from build123d import *

# Parameters (mm, degrees)
EXTRUDE004_DEPTH                     = 120
EXTRUDE004_ONTO_SKETCH004_ROLL_ANGLE = 90
ARRAY005_X_COUNT                     = 2
ARRAY005_X_PITCH                     = 51
EXTRUDE001_DEPTH                     = 120
EXTRUDE001_ONTO_SKETCH001_ROLL_ANGLE = 90
ARRAY003_Z_COUNT                     = 2
ARRAY003_Z_PITCH                     = 21
EXTRUDE003_DEPTH                     = 119
EXTRUDE003_ONTO_SKETCH003_ROLL_ANGLE = 90
ARRAY_X_COUNT                        = 2
ARRAY_X_PITCH                        = 51
EXTRUDE002_DEPTH                     = 119
EXTRUDE002_ONTO_SKETCH002_ROLL_ANGLE = 90
ARRAY004_Z_COUNT                     = 2
ARRAY004_Z_PITCH                     = 21
BOX002_W                             = 96
BOX002_H                             = 118
BOX002_DEPTH                         = 1
BOX001_W                             = 96
BOX001_H                             = 118
BOX001_DEPTH                         = 41
BOX_W                                = 102
BOX_H                                = 120
BOX_DEPTH                            = 47
EXTRUDE_DEPTH                        = 0.8
ARRAY002_X_COUNT                     = 8
ARRAY002_X_PITCH                     = 12
ARRAY002_Z_COUNT                     = 2
ARRAY002_Z_PITCH                     = 21
FILLET_R                             = 0.5


with BuildPart() as bottomsideguidearray:
    # Sketch004 as drawn → Extrude004 (new)
    with BuildSketch(Plane.XY):
        Polygon((-6, 1), (4, 1), (2, -1), (-4, -1), align=None)
    extrude(amount=-EXTRUDE004_DEPTH)


with BuildPart() as bottomsideguidearray_1:
    # Extrude004 onto Sketch004 roll: moved
    add(bottomsideguidearray.part.rotate(Axis((0, 0, 0), (1, 0, 0)), EXTRUDE004_ONTO_SKETCH004_ROLL_ANGLE))


with BuildPart() as bottomsideguidearray_2:
    # Extrude004 onto Sketch004 placement: moved
    add(bottomsideguidearray_1.part)


with BuildPart() as bottomsideguidearray_3:
    # Extrude004 placement: moved
    add(bottomsideguidearray_2.part.moved(Location((25.5, 0, 0))))

    # Array005 X: BottomSideGuideArray ×2


with BuildPart() as bottomsideguidearray_4:
    add(bottomsideguidearray_3.part)
    with Locations(*[(i * ARRAY005_X_PITCH, 0, 0) for i in range(1, ARRAY005_X_COUNT)]):
        add(bottomsideguidearray_3.part)


with BuildPart() as guidegaps:
    # Sketch001 as drawn → Extrude001 (new)
    with BuildSketch(Plane.XY):
        Polygon((0, 0), (0, 10), (2, 8), (2, 2), align=None)
    extrude(amount=-EXTRUDE001_DEPTH)


with BuildPart() as guidegaps_1:
    # Extrude001 onto Sketch001 roll: moved
    add(guidegaps.part.rotate(Axis((0, 0, 0), (1, 0, 0)), EXTRUDE001_ONTO_SKETCH001_ROLL_ANGLE))


with BuildPart() as guidegaps_2:
    # Extrude001 onto Sketch001 placement: moved
    add(guidegaps_1.part.moved(Location((99, 0, 7))))

    # Array003 Z: GuideGaps ×2


with BuildPart() as guidegaps_3:
    add(guidegaps_2.part)
    with Locations(*[(0, 0, i * ARRAY003_Z_PITCH) for i in range(1, ARRAY003_Z_COUNT)]):
        add(guidegaps_2.part)

    # Fusion003: union BottomSideGuideArray
    add(bottomsideguidearray_4.part)


with BuildPart() as topsideguidearray:
    # Sketch003 as drawn → Extrude003 (new)
    with BuildSketch(Plane.XY):
        Polygon((-5.2, 47.6), (3.2, 47.6), (1.6, 46), (-3.6, 46), align=None)
    extrude(amount=-EXTRUDE003_DEPTH)


with BuildPart() as topsideguidearray_1:
    # Extrude003 onto Sketch003 roll: moved
    add(topsideguidearray.part.rotate(Axis((0, 0, 0), (1, 0, 0)), EXTRUDE003_ONTO_SKETCH003_ROLL_ANGLE))


with BuildPart() as topsideguidearray_2:
    # Extrude003 onto Sketch003 placement: moved
    add(topsideguidearray_1.part)


with BuildPart() as topsideguidearray_3:
    # Extrude003 placement: moved
    add(topsideguidearray_2.part.moved(Location((25.5, 1, 0))))

    # Array X: TopSideGuideArray ×2


with BuildPart() as topsideguidearray_4:
    add(topsideguidearray_3.part)
    with Locations(*[(i * ARRAY_X_PITCH, 0, 0) for i in range(1, ARRAY_X_COUNT)]):
        add(topsideguidearray_3.part)


with BuildPart() as guiderods:
    # Sketch002 as drawn → Extrude002 (new)
    with BuildSketch(Plane.XY):
        Polygon((0.4, 9.2), (0.4, 0.8), (2, 2.4), (2, 7.6), align=None)
    extrude(amount=-EXTRUDE002_DEPTH)


with BuildPart() as guiderods_1:
    # Extrude002 onto Sketch002 roll: moved
    add(guiderods.part.rotate(Axis((0, 0, 0), (1, 0, 0)), EXTRUDE002_ONTO_SKETCH002_ROLL_ANGLE))


with BuildPart() as guiderods_2:
    # Extrude002 onto Sketch002 placement: moved
    add(guiderods_1.part.moved(Location((-1, 0, 7))))


with BuildPart() as guiderods_3:
    # Extrude002 placement: moved
    add(guiderods_2.part.moved(Location((-2, 1, 0))))

    # Array004 Z: GuideRods ×2


with BuildPart() as guiderods_4:
    add(guiderods_3.part)
    with Locations(*[(0, 0, i * ARRAY004_Z_PITCH) for i in range(1, ARRAY004_Z_COUNT)]):
        add(guiderods_3.part)

    # Fusion002: union TopSideGuideArray
    add(topsideguidearray_4.part)


with BuildPart() as separator:
    # Box002 → Box002 (new body)
    with BuildSketch(Plane(origin=(2, 0, 22), x_dir=(1, 0, 0), z_dir=(0, 0, 1))):
        with Locations((48, 59)):
            Rectangle(BOX002_W, BOX002_H)
    extrude(amount=BOX002_DEPTH)


with BuildPart() as inner_box:
    # Box001 → Box001 (new body)
    with BuildSketch(Plane(origin=(2, 0, 2), x_dir=(1, 0, 0), z_dir=(0, 0, 1))):
        with Locations((48, 59)):
            Rectangle(BOX001_W, BOX001_H)
    extrude(amount=BOX001_DEPTH)


with BuildPart() as cabinet_base:
    # Box → Box (new body)
    with BuildSketch(Plane(origin=(-1, 0, -1), x_dir=(1, 0, 0), z_dir=(0, 0, 1))):
        with Locations((51, 60)):
            Rectangle(BOX_W, BOX_H)
    extrude(amount=BOX_DEPTH)

    # Cut: cut Inner Box
    add(inner_box.part, mode=Mode.SUBTRACT)

    # Fusion: union Separator
    add(separator.part)


with BuildPart() as final_cabinet:
    # Sketch → Extrude (new body)
    with BuildSketch(Plane.XY):
        Polygon((0.5, 0), (0.25, 104), (0.25, 105), (1.75, 105), (1.75, 104), (1.5, 0), align=None)
    extrude(amount=EXTRUDE_DEPTH)

    # Array002 X: Final Cabinet ×8


with BuildPart() as final_cabinet_1:
    add(final_cabinet.part)
    with Locations(*[(i * ARRAY002_X_PITCH, 0, 0) for i in range(1, ARRAY002_X_COUNT)]):
        add(final_cabinet.part)

    # Array002 Z: Final Cabinet ×2


with BuildPart() as final_cabinet_2:
    add(final_cabinet_1.part)
    with Locations(*[(0, 0, i * ARRAY002_Z_PITCH) for i in range(1, ARRAY002_Z_COUNT)]):
        add(final_cabinet_1.part)


with BuildPart() as final_cabinet_3:
    # Array002 placement: moved
    add(final_cabinet_2.part.moved(Location((7, 13, 2))))

    # Fusion001: union Cabinet Base
    add(cabinet_base.part)

    # Fillet
    fillet_edges = [final_cabinet_3.edges().sort_by_distance(p)[0] for p in [
        (-1, 0, 22.5),
        (-1, 60, 46),
        (-1, 120, 22.5),
        (-1, 60, -1),
        (50, 0, -1),
        (101, 0, 22.5),
        (50, 0, 46),
        (50, 120, 46),
        (101, 60, 46),
        (50, 120, -1),
        (101, 120, 22.5),
        (101, 60, -1),
    ]]
    fillet(fillet_edges, radius=FILLET_R)

    # Fusion004: union GuideRods
    add(guiderods_4.part)

    # Cut001: cut GuideGaps
    add(guidegaps_3.part, mode=Mode.SUBTRACT)


solid = final_cabinet_3.part
Geometry check sheet. Reference: the model listing, model coordinates, mm. A direction names the side the tool comes from. Give positions to 0.01 mm unless a question says otherwise; leave off trailing zeros. Write each loop counter-clockwise with the first axis right and the second up, starting at its lowest first coordinate (ties: lowest second). Pieces come first, ordered by that corner, then holes. Notation, with made-up numbers: M -15,-28 L -3,-28 A13 cw -3,-4 Z; hole C 36.25,30 d6. An arc over 180 degrees is marked long. Answer as CSV lines item,"result". Start each with the question number.
Q1. Section check D-D, the plane z = 20. Record the cut outline in (x, y).
Q2. Section check C-C, the plane y = 8. Give the number of separate pieces and of enclosed holes in the cut face, then the cut area to 3 significant figures.
Q3. Tool access check on faces 1 (the face through (24, 59, 1)), 2 (the face through (24, 60, 47.6)), 3 (the face through (49, 60, 22)). Record the directions out of +Z, -Z, +X, -X, +Y, -Y that give a thin tool (end or side, any length) a straight path to the whole face; none if there is none.
Q4. Material ranges on L1, parallel to Z at x = 94.5, y = 87; L2, parallel to X at y = 114, z = 16; L3, parallel to X at y = 108.5, z = 33, recorded low to high.
Q5. Go/stop test with flat-tipped pins: pin 1 (6 mm diameter, centred on x = 31.5, z = 33.5, fed in from -Y); pin 2 (2 mm diameter, centred on x = 75, y = 40.5, fed in from -Z); pin 3 (0.9 mm diameter, centred on x = 80, z = 2.5, fed in from -Y). Record where each tip stops, or that it passes through.
Q6. Section check A-A, the plane z = 11. Record the cut outline in (x, y).
Q7. Release check for a two-part mould opening along X. For faces 4 (the face through (-2.6, 60, 33)), 5 (the face through (101, 59, 41)), 6 (the face through (99, 59, 12)) record: pulls with the +X half, pulls with the -X half, needs draft (parallel to the pull), parting line crosses it, or undercut.
Q8. Section check B-B, the plane x = 60.5. Record the cut outline in (y, z), then the cut area to 3 significant figures.
Geometry says:
1,outline,"M -1,0.5 A0.5 ccw -0.5,0 L 2,0 L 2,118 L 98,118 L 98,0 L 100.5,0 A0.5 ccw 101,0.5 L 101,119.5 A0.5 ccw 100.5,120 L -0.5,120 A0.5 ccw -1,119.5 Z"
2,separate pieces,"1"
2,enclosed holes,"2"
2,area,"933 mm^2"
3,face 1,"+Y, -Y"
3,face 2,"+Z, +X, -X, +Y, -Y"
3,face 3,"-Y"
4,L1,"-1 to 2, 22 to 23, 43 to 46"
4,L2,"-2.6 to -2.4, -1 to 2, 98 to 99, 100 to 101"
4,L3,"-2.6 to 2, 98 to 99"
5,pin 1,"y = 118"
5,pin 2,"z = 1"
5,pin 3,"y = 13"
6,outline,"M -2.6,1 L -1,1 L -1,0.5 A0.5 ccw -0.5,0 L 2,0 L 2,118 L 98,118 L 98,0 L 99,0 L 99,120 L -0.5,120 A0.5 ccw -1,119.5 L -1,120 L -2.6,120 Z"
7,face 4,"pulls with the -X half"
7,face 5,"pulls with the +X half"
7,face 6,"undercut"
8,outline,"M 0,-0.5 A0.5 ccw 0.5,-1 L 119.5,-1 A0.5 ccw 120,-0.5 L 120,45.5 A0.5 ccw 119.5,46 L 0.5,46 A0.5 ccw 0,45.5 L 0,43 L 118,43 L 118,23 L 0,23 L 0,22 L 118,22 L 118,2 L 0,2 Z"
8,area,"920 mm^2"
